Input: part model. Units: mm. Frame: model coordinates. A direction names the side the tool comes from. Coordinates: 2 decimals unless noted, no trailing zeros. Order: outer loops, then holes, each group sorted by start corner. A loop starts at its lowest first (then second) coordinate and runs counter-clockwise, first axis right, second up. Notation, with made-up numbers: (-13.75, 45) -> (28.25, 45) arc R26 cw to (28.25, 60) -> close; hole circle Ø11 at (-12.75, 52.5). An arc over 180 degrees is marked (long way). Use one line per item in the form item = value. Start each with the question number.
1) Access query for faces 1 (the flat face through (6.453, -0.28, 6.275)), 2 (the flat face through (-42, 0, -20)), 3 (the flat face through (-43, 0, 20)), 4 (the flat face through (-7, -10, 15)). Directions: +Z, -Z, +X, -X, +Y, -Y. A direction counts if a zero-diameter tool reaches every point of the face in a straight line with its end or side. Return the directions, or none.
2) Section query C-C on x = -24. Output: boundary loops of the cut face in (y, z).
3) Section query D-D on y = -12.5. Output: boundary loops of the cut face in (x, z).
4) Pin query (flat end, axial travel): pin 1 (18.5 mm diameter, centred on x = -35, y = 4, fed in from -Z); pin 2 (11 mm diameter, centred on y = 9.5, z = 46.5, fed in from -X); pin 3 (8 mm diameter, centred on x = 30, z = 10.5, fed in from +Y). Return the tip coordinate at first contact, or that it passes through.
5) Section query A-A on y = 15. Output: boundary loops of the cut face in (x, z), then the cut area to 3 significant figures.
6) Section query B-B on y = 7. Output: boundary loops of the cut face in (x, z).
7) Ray query, line 1 along X through (y, z) = (2.5, -32); line 2 along Y through (x, z) = (-12.5, 26). Return the intervals inside material, ascending.
from build123d import *

# Parameters (mm, degrees)
F3_DEPTH = 40.001
F5_DEPTH = 40.0010001


with BuildPart() as f1:
    # F0 (on Top) → F1 (revolve)
    with BuildSketch(Plane.XY):
        with BuildLine():
            Line((-60, 20), (-60, 10))
            Line((-60, 10), (-60, -10))
            Line((-60, -10), (-60, -20))
            Line((-60, -20), (-52, -20))
            ThreePointArc((-52, -20), (-45.3623174839, -12.7029414592), (-35.8754845034, -10))
            Line((-35.8754845034, -10), (-16, -10))
            Line((-16, -10), (-16, -20))
            Line((-16, -20), (0, -20))
            Line((0, -20), (0, 20))
            Line((0, 20), (-16, 20))
            Line((-16, 20), (-16, 10))
            Line((-16, 10), (-35.8754845034, 10))
            ThreePointArc((-35.8754845034, 10), (-45.3623174839, 12.7029414592), (-52, 20))
            Line((-52, 20), (-60, 20))
        make_face()
    revolve(axis=Axis((0, 0.0902060419, 0), (0, -1, 0)))

    # F2 (on face) → F3 (cut, through all)
    with BuildSketch(Plane.XZ.offset(20)):
        with BuildLine():
            Line((48, 20), (56.5685424949, 20))
            ThreePointArc((56.5685424949, 20), (42.4264068712, 42.4264068712), (20, 56.5685424949))
            Line((20, 56.5685424949), (20, 48))
            ThreePointArc((20, 48), (36.7695526217, 36.7695526217), (48, 20))
        make_face()
        with BuildLine():
            Line((20, 20), (48, 20))
            ThreePointArc((48, 20), (36.7695526217, 36.7695526217), (20, 48))
            Line((20, 48), (20, 20))
        make_face()
        with BuildLine():
            Line((-20, 20), (-20, 48))
            ThreePointArc((-20, 48), (-36.7695526217, 36.7695526217), (-48, 20))
            Line((-48, 20), (-20, 20))
        make_face()
        with BuildLine():
            Line((-20, 48), (-20, 56.5685424949))
            ThreePointArc((-20, 56.5685424949), (-42.4264068712, 42.4264068712), (-56.5685424949, 20))
            Line((-56.5685424949, 20), (-48, 20))
            ThreePointArc((-48, 20), (-36.7695526217, 36.7695526217), (-20, 48))
        make_face()
        with BuildLine():
            ThreePointArc((-56.5685424949, -20), (-42.4264068712, -42.4264068712), (-20, -56.5685424949))
            Line((-20, -56.5685424949), (-20, -48))
            ThreePointArc((-20, -48), (-36.7695526217, -36.7695526217), (-48, -20))
            Line((-48, -20), (-56.5685424949, -20))
        make_face()
        with BuildLine():
            ThreePointArc((-48, -20), (-36.7695526217, -36.7695526217), (-20, -48))
            Line((-20, -48), (-20, -20))
            Line((-20, -20), (-48, -20))
        make_face()
        with BuildLine():
            ThreePointArc((20, -56.5685424949), (42.4264068712, -42.4264068712), (56.5685424949, -20))
            Line((56.5685424949, -20), (48, -20))
            ThreePointArc((48, -20), (36.7695526217, -36.7695526217), (20, -48))
            Line((20, -48), (20, -56.5685424949))
        make_face()
        with BuildLine():
            ThreePointArc((20, -48), (36.7695526217, -36.7695526217), (48, -20))
            Line((48, -20), (20, -20))
            Line((20, -20), (20, -48))
        make_face()
    extrude(amount=-F3_DEPTH, mode=Mode.SUBTRACT)

    # F4 (on face) → F5 (cut, through all)
    with BuildSketch(Plane.XZ.offset(20)):
        Polygon((0, -12.7279), (12.7279, 0), (0, 12.7279), (-12.7279, 0), align=None)
    extrude(amount=-F5_DEPTH, mode=Mode.SUBTRACT)


solid = f1.part
Answers below:
q1.face_1 = +Y, -Y
q1.face_2 = -Z, -X, +Y, -Y
q1.face_3 = +Z, -X, +Y, -Y
q1.face_4 = -Y
q2.outline = (-10, -20) -> (10, -20) -> (10, 20) -> (-10, 20) -> close
q3.outline = (-56.57, -20) -> (-40.34, -20) arc R45.03 cw to (-40.34, 20) -> (-56.57, 20) arc R60 ccw to start; (-20, -56.57) arc R60 ccw to (20, -56.57) -> (20, -40.34) arc R45.03 cw to (-20, -40.34) -> close; (-20, 40.34) arc R45.03 cw to (20, 40.34) -> (20, 56.57) arc R60 ccw to (-20, 56.57) -> close; circle Ø32 at (0, 0); (40.34, -20) -> (56.57, -20) arc R60 ccw to (56.57, 20) -> (40.34, 20) arc R45.03 cw to start; hole (-12.73, 0) -> (0, -12.73) -> (12.73, 0) -> (0, 12.73) -> close
q4.pin_1 = -20
q4.pin_2 = -20
q4.pin_3 = 10
q5.outline = (-56.57, -20) -> (-43.99, -20) arc R48.33 cw to (-43.99, 20) -> (-56.57, 20) arc R60 ccw to start; (-20, -56.57) arc R60 ccw to (20, -56.57) -> (20, -43.99) arc R48.33 cw to (-20, -43.99) -> close; (-20, 43.99) arc R48.33 cw to (20, 43.99) -> (20, 56.57) arc R60 ccw to (-20, 56.57) -> close; circle Ø32 at (0, 0); (43.99, -20) -> (56.57, -20) arc R60 ccw to (56.57, 20) -> (43.99, 20) arc R48.33 cw to start; hole (-12.73, 0) -> (0, -12.73) -> (12.73, 0) -> (0, 12.73) -> close
q5.area = 2,390 mm^2
q6.outline = (-56.57, -20) -> (-20, -20) -> (-20, -56.57) arc R60 ccw to (20, -56.57) -> (20, -20) -> (56.57, -20) arc R60 ccw to (56.57, 20) -> (20, 20) -> (20, 56.57) arc R60 ccw to (-20, 56.57) -> (-20, 20) -> (-56.57, 20) arc R60 ccw to start; hole (-12.73, 0) -> (0, -12.73) -> (12.73, 0) -> (0, 12.73) -> close
q7.line_1 = -20 to 20
q7.line_2 = -10 to 10
